For this review, take the finished solid that the model builds, in its own axes (mm). A direction names the side the tool comes from. Round coordinates to 2 decimals unless told otherwise and drop trailing zeros. Order: outer loops, then holes, each group sorted by start corner. A loop starts at its lowest first (then second) coordinate and runs counter-clockwise, first axis right, second up. Notation, with made-up numbers: (2, -12) - (40, -12) arc R29 ccw to (40, 23) - close; hole circle Ø7 at (-27.75, 70). An arc over 180 degrees is marked (long way). One line per item, written item: value.
Autodesk Inventor part; units mm, degrees
ref_plane "YZ Plane" through (0, 0, 0) normal (1, 0, 0) x (0, 1, 0)
ref_plane "XZ Plane" through (0, 0, 0) normal (0, 1, 0) x (-1, 0, 0)
ref_plane "XY Plane" through (0, 0, 0) normal (0, 0, 1) x (1, 0, 0)
sketch "スケッチ1" plane through (0, 0, 0) normal (0, 1, 0) x (-1, 0, 0)
  circle A0 centre (0, 0) radius 16
  dimension "d0" = 32
extrude "押し出し1" add sketch "スケッチ1" along normal blind 20
sketch "スケッチ2" plane through (0, 20, 0) normal (0, 1, 0) x (1, 0, 0)
  circle A0 centre (0, 0) radius 13
  dimension "d3" = 26
extrude "押し出し2" add sketch "スケッチ2" along normal blind 10
sketch "スケッチ3" plane through (0, 30, 0) normal (0, 1, 0) x (1, 0, 0)
  arc A0 (-8.6603, 5) -> (-10, 0) centre (0, 0) ccw
  line L0 (0, 0) -> (-8.6603, 5) construction
  line L1 (0, 0) -> (-10, 0) construction
  arc A1 (-5.5063, 7.8639) -> (-8.3138, 4.8) centre (0, 0) ccw
  line L2 (0, 0) -> (-5.5063, 7.8639) construction
  line L3 (0, 0) -> (-8.3138, 4.8) construction
  arc A2 (8.6603, -5) -> (10, 0) centre (0, 0) ccw
  line L4 (0, 0) -> (8.6603, -5) construction
  line L5 (0, 0) -> (10, 0) construction
  arc A3 (5.5063, -7.8639) -> (8.3138, -4.8) centre (0, 0) ccw
  line L6 (0, 0) -> (5.5063, -7.8639) construction
  line L7 (0, 0) -> (8.3138, -4.8) construction
  line L8 (-8.6603, 5) -> (-8.3138, 4.8)
  line L9 (8.6603, -5) -> (8.3138, -4.8)
  line L10 (-5.5063, 7.8639) -> (5.5063, -7.8639)
  line L11 (-10, 0) -> (10, 0)
  dimension "d6" = 10
  dimension "d7" = 30
  dimension "d10" = 9.6
  dimension "d11" = 25
  dimension "d12" = 10
  dimension "d13" = 30
  dimension "d14" = 9.6
  dimension "d15" = 25
extrude "押し出し3" add sketch "スケッチ3" along normal blind 5
fillet "フィレット1" radius 1 2 edges at (-5.5063, 32.5, -7.8639) (5.5063, 32.5, 7.8639)
sketch "スケッチ4" plane through (0, 35, 0) normal (0, 1, 0) x (1, 0, 0)
  line L0 (-4.8993, 6.9969) -> (0, 0)
  line L1 (4.8993, -6.9969) -> (0, 0)
  arc A0 (7.4565, -10.649) -> (13, 0) centre (0, 0) ccw
  line L2 (0, 0) -> (7.4565, -10.649) construction
  line L3 (0, 0) -> (13, 0) construction
  line L4 (0, 0) -> (10, 0)
  arc A1 (-7.4565, 10.649) -> (-13, 0) centre (0, 0) ccw
  line L5 (0, 0) -> (-7.4565, 10.649) construction
  line L6 (0, 0) -> (-13, 0) construction
  circle A2 centre (0, 0) radius 13
  line L7 (7.4565, -10.649) -> (0, 0)
  line L8 (0, 0) -> (13, 0)
  line L9 (0, 0) -> (-13, 0)
  line L10 (0, 0) -> (-7.4565, 10.649)
  dimension "d21" = 13
  dimension "d22" = 55
  dimension "d23" = 13
  dimension "d24" = 55
extrude "押し出し4" add sketch "スケッチ4" along normal blind 2 contours L0 L9 A1 L10 | L4 L8 A0 L7 L1
properties part number "kumi4-1"
Item 1: Take a section at C-C (y = 14). Write out the cut boundary in (x, z), plus the area to 3 significant figures.
Returned:
outline: circle Ø32 at (0, 0)
area: 804 mm^2
Item 2: Take a section at B-B (x = 11.5). Write out the cut boundary in (y, z), plus the area to 3 significant figures.
Returned:
outline: (0, -11.12) - (20, -11.12) - (20, -6.06) - (30, -6.06) - (30, 6.06) - (20, 6.06) - (20, 11.12) - (0, 11.12) - close; (35, 0) - (37, 0) - (37, 6.06) - (35, 6.06) - close
area: 578 mm^2
Item 3: Wall thickness on line 1 (Y direction, x = -8, z = -9); line 2 (Y direction, x = 3.5, z = 11.5); line 3 (Z direction, x = 0, y = 2): over which ranges is each line inside the solid? List them lowest first.
Returned:
line 1: 0 to 30, 35 to 37
line 2: 0 to 30
line 3: -16 to 16
Item 4: The part is to be moulded in two halves that separate along Y. For faces 4 (the cylindrical face through (5.591, 32.535, 7.415)), 5 (the flat face through (-2.484, 32.465, -3.547)), 6 (the flat face through (-8, 37, -4)), 7 (the flat face through (0, 0, 0)), say which applies: +Y half, -Y half, draft (parallel to the pull), parting line (faces both ways), or undercut.
Returned:
face 4: undercut
face 5: draft
face 6: +Y half
face 7: -Y half
Item 5: For P1, Ø2, axis at x = 10, y = 17.5, coming from the -Z side; P2, Ø1.5, axis at x = -1.5, y = 29.5, coming from the +Z side; P3, Ø1, axis at x = -0.5, y = 12.5, coming from the -Z side; P4, Ø2, axis at x = -5, y = 20, coming from the +Z side, all flat-tipped, find the tip position at first contact; note any pin that passes through.
Returned:
P1: z = -13.23
P2: z = 12.98
P3: z = -16
P4: z = 15.49
Item 6: Machinability: for faces 1 (the flat face through (-5, 33, 0)), 2 (the cylindrical face through (-11.57, 35.99, -5.93)), 3 (the cylindrical face through (9.67, 32.47, 2.55)), which of the approach directions +Z, -Z, +X, -X, +Y, -Y give a long, thin tool a straight path to every point of the face, cutting with its end or side? Answer none if there is none.
Returned:
face 1: +Z, -X, +Y
face 2: -Z, -X, +Y
face 3: +Z, +X
Item 7: Take a section at A-A (z = -8.5). Write out the cut boundary in (x, y), plus the area to 3 significant figures.
Returned:
outline: (-13.56, 0) - (13.56, 0) - (13.56, 20) - (9.84, 20) - (9.84, 30) - (-9.84, 30) - (-9.84, 20) - (-13.56, 20) - close; (-9.84, 35) - (-5.95, 35) - (-5.95, 37) - (-9.84, 37) - close
area: 747 mm^2
